Here's how the part is built. I have some questions about the finished solid (model axes, mm). A direction names the side the tool comes from. Round coordinates to 2 decimals unless told otherwise and drop trailing zeros. Write each loop counter-clockwise with the first axis right and the second up, starting at its lowest first coordinate (ties: lowest second). Pieces come first, ordered by that corner, then holes. Notation, with made-up numbers: (-6.75, -34) -> (44.25, -34) arc R7 ccw to (44.25, -25) -> close; hole circle Ø5 at (21, 53). An arc over 180 degrees is marked (long way). Answer as CSV lines item,"result".
Autodesk Inventor part; units mm, degrees
ref_plane "YZ Plane" through (0, 0, 0) normal (1, 0, 0) x (0, 1, 0)
ref_plane "XZ Plane" through (0, 0, 0) normal (0, 1, 0) x (-1, 0, 0)
ref_plane "XY Plane" through (0, 0, 0) normal (0, 0, 1) x (1, 0, 0)
sketch "Sketch1" plane through (0, 0, 0) normal (1, 0, 0) x (0, 1, 0)
  circle A0 centre (0, 0) radius 8
  circle A1 centre (0, 0) radius 6.35
  dimension "d0" = 16
  dimension "d3" = 12.7
extrude "Extrusion1" add sketch "Sketch1" along normal mid plane 420 contours A1
extrude "Extrusion2" add sketch "Sketch1" along normal mid plane 260
thread "Thread1"
properties part number "driveshaft1"
1. Suppose I cut it at C-C on x = 164.5. Please give me the cut outline in (y, z).
Numbers:
outline,"circle Ø12.7 at (0, 0)"
2. Suppose I cut it at D-D on x = 11. Please give me the cut outline in (y, z), and give its area (3 significant figures).
Numbers:
outline,"circle Ø16 at (0, 0)"
area,"201 mm^2"
3. If I drill on line 1 (Z direction, x = 165.5, y = 0.5); line 2 (Y direction, x = -188, z = 0.75); line 3 (Z direction, x = -63, y = -0.5), over which ranges is the centre line in solid material (lowest first)?
Numbers:
line 1,"z = -6.33 to 6.33"
line 2,"y = -6.31 to 6.31"
line 3,"z = -7.98 to 7.98"
4. Suppose I cut it at A-A on z = 0. Please give me the cut outline in (x, y), and give its area (3 significant figures).
Numbers:
outline,"(-210, -6.35) -> (-130, -6.35) -> (-130, -8) -> (130, -8) -> (130, -6.35) -> (210, -6.35) -> (210, 6.35) -> (130, 6.35) -> (130, 8) -> (-130, 8) -> (-130, 6.35) -> (-210, 6.35) -> close"
area,"6,190 mm^2"
5. For pin 1 Ø1.5 at (x, y) = (10.5, 1) entering from +Z; pin 2 Ø2 at (x, z) = (56.5, -6) entering from +Y (3 decimals), each with a flat end and sliding along its axis, tell me the tip position at first contact or that it passes through.
Numbers:
pin 1,"stops at z = 8"
pin 2,"stops at y = 6.245"
6. On a 3-axis mill with a long thin cutter (end or side, diameter ignored), from which of +Z, -Z, +X, -X, +Y, -Y can I reach the whole of each face in a straight line? I mean faces 1 (the face through (-169.44, -1.38, -6.2)), 2 (the face through (169.44, -1.38, 6.2)), 3 (the face through (1.82, -1.73, -7.81)). Say none if no direction works.
Numbers:
face 1,"-X"
face 2,"+X"
face 3,"+X, -X"
